Autodesk Inventor part; units mm, degrees
ref_plane "YZ Plane" through (0, 0, 0) normal (1, 0, 0) x (0, 1, 0)
ref_plane "XZ Plane" through (0, 0, 0) normal (0, 1, 0) x (-1, 0, 0)
ref_plane "XY Plane" through (0, 0, 0) normal (0, 0, 1) x (1, 0, 0)
sketch "Sketch1" plane through (0, 0, 0) normal (0, 1, 0) x (-1, 0, 0)
  circle A0 centre (0, 0) radius 2.5
  circle A1 centre (0, 0) radius 8.95
  circle A2 centre (0, 0) radius 6.1
  dimension "d0" = 5
  dimension "d1" = 17.9
  dimension "d2" = 12.2
extrude "Extrusion1" add sketch "Sketch1" along normal blind 1 contours A1 | A2
extrude "Extrusion2" add sketch "Sketch1" along normal blind 7.6 contours A2
sketch "Sketch2" plane through (0, 7.6, 0) normal (0, 1, 0) x (1, 0, 0)
  circle A0 centre (0, 0) radius 8.95
  circle A1 centre (0, 0) radius 2.5
extrude "Extrusion3" add sketch "Sketch2" along normal blind 1
sketch "Sketch3" plane through (0, 0, 0) normal (0, -1, 0) x (1, 0, 0)
  circle A0 centre (0, 0) radius 3
  circle A1 centre (0, 0) radius 3.25
  dimension "d9" = 6
  dimension "d10" = 6.5
sketch "Sketch4" plane through (0, 8.6, 0) normal (0, 1, 0) x (1, 0, 0)
  circle A0 centre (0, 0) radius 3
  circle A1 centre (0, 0) radius 3.25
  dimension "d11" = 6
  dimension "d12" = 6.5
extrude "Extrusion4" cut sketch "Sketch4" against normal blind 0.5
extrude "Extrusion5" cut sketch "Sketch3" against normal blind 0.5
properties part number "Wheel"
CAD build for the part. Positions are in the model's coordinates, mm. A direction names the side the tool comes from. Give positions to 0.01 mm unless a question says otherwise; leave off trailing zeros. Order: outer loops, then holes, each group sorted by start corner. A loop starts at its lowest first (then second) coordinate and runs counter-clockwise, first axis right, second up. Notation, with made-up numbers: M 9.25,68 L 47.25,68 A32 ccw 47.25,97 Z; hole C 81.25,51 d4. An arc over 180 degrees is marked long. Put each result on its own line as item: value. Start each with the question number.
(1) Saw through at B-B, the plane z = -7. Write the cut outline in (x, y).
(2) Which spindle directions (+Z, -Z, +X, -X, +Y, -Y) get a long thin tool onto all of the face, cutting with end or side? Do faces 1 (the cylindrical face through (-3, 0.2, 0.1)), 2 (the flat face through (2, 7.6, 6)), 3 (the flat face through (2, 0, 2)), 4 (the cylindrical face through (7.1, 0.49, 5.45)), 5 (the cylindrical face through (-2.579, 8.354, 1.978)). Say none if no direction does.
(3) Mould opens along Z. For faces 6 (the flat face through (-2, 8.6, -2)), 7 (the cylindrical face through (-2.579, 0.246, -1.978)), 8 (the cylindrical face through (6.094, 4.254, -0.268)), 9 (the cylindrical face through (-3, 8.4, -0.1)) say: +Z half, -Z half, draft (parallel to the pull), parting line (faces both ways), or undercut.
(4) Saw through at C-C, the plane y = 6. Write the cut outline in (x, z), then the cut area to 3 significant figures.
(5) Drill centre lines: line 1 along Z through (x, y) = (0, 8.3); line 2 along X through (y, z) = (2.5, 0). Where is each one in solid material? Low to high.
(6) Saw through at D-D, the plane z = 5.25. Write the cut outline in (x, y), then the cut area to 3 significant figures.
Check result:
1. outline: M -5.58,0 L 5.58,0 L 5.58,1 L -5.58,1 Z; M -5.58,7.6 L 5.58,7.6 L 5.58,8.6 L -5.58,8.6 Z
2. face 1: -Y
2. face 2: none
2. face 3: +Z, -Z, +X, -X, -Y
2. face 4: +Y, -Y
2. face 5: +Y
3. face 6: draft
3. face 7: undercut
3. face 8: parting line
3. face 9: undercut
4. outline: C 0,0 d12.2; hole C 0,0 d5
4. area: 97.3 mm2
5. line 1: z = -8.95 to -3.25, -3 to -2.5, 2.5 to 3, 3.25 to 8.95
5. line 2: x = -6.1 to -2.5, 2.5 to 6.1
6. outline: M -7.25,0 L 7.25,0 L 7.25,1 L 3.11,1 L 3.11,7.6 L 7.25,7.6 L 7.25,8.6 L -7.25,8.6 L -7.25,7.6 L -3.11,7.6 L -3.11,1 L -7.25,1 Z
6. area: 70.0 mm2
